Work out the finished part from the listing and answer in its coordinate system (mm). A direction names the side the tool comes from. Give positions to 0.01 mm unless a question says otherwise; leave off trailing zeros. Loops run counter-clockwise (first coordinate to the right, second up) from the corner with the lowest first, then second, coordinate; pieces in that order, holes last. Notation, with made-up numbers: (-22, 59.5) - (10, 59.5) arc R16 cw to (10, 88.5) - close; hole circle Ø9 at (38, 59). An arc over 180 degrees is marked (long way). Use CSV: the item, a comma, the result in double quotes.
Autodesk Inventor part; units mm, degrees
ref_plane "YZ Plane" through (0, 0, 0) normal (1, 0, 0) x (0, 1, 0)
ref_plane "XZ Plane" through (0, 0, 0) normal (0, 1, 0) x (-1, 0, 0)
ref_plane "XY Plane" through (0, 0, 0) normal (0, 0, 1) x (1, 0, 0)
sketch "Sketch1" plane through (0, 0, 0) normal (1, 0, 0) x (0, 1, 0)
  line L0 (10.236, 20.6024) -> (1.9777, 20.6024)
  line L1 (1.9777, 20.6024) -> (1.9777, 4.6508)
  line L2 (1.9777, 4.6508) -> (10.236, 4.6508)
  line L3 (10.236, 4.6508) -> (10.236, 20.6024)
  point P0 (0, 0)
extrude "Extrusion1" add sketch "Sketch1" along normal blind 25.4
sketch "Sketch2" plane through (0, 10.236, 20.6024) normal (0, 1, 0) x (1, 0, 0)
  line L0 (6.7613, 3.64) -> (20.9369, 3.64)
  line L1 (20.9369, 3.64) -> (20.9369, 12.1675)
  line L2 (20.9369, 12.1675) -> (6.7613, 12.1675)
  line L3 (6.7613, 12.1675) -> (6.7613, 3.64)
  line L4 (10.89, 6.1434) -> (17.4809, 6.1434)
  line L5 (17.4809, 6.1434) -> (17.4809, 9.7454)
  line L6 (17.4809, 9.7454) -> (11.2732, 9.7454)
  line L7 (11.2732, 9.7454) -> (11.2732, 6.1434)
  point P0 (0, 20.6024)
extrude "Extrusion2" add sketch "Sketch2" along normal blind 25.4 contours L3 L2 L1 L0 | L7 L6 L5 L4
sketch "Sketch3" plane through (0, 35.636, 20.6024) normal (0, 1, 0) x (1, 0, 0)
  line L0 (10.6145, 6.041) -> (18.3551, 6.041)
  line L1 (18.3551, 6.041) -> (18.3551, 10.1795)
  line L2 (18.3551, 10.1795) -> (10.6145, 10.1795)
  line L3 (10.6145, 10.1795) -> (10.6145, 6.041)
  point P0 (0, 20.6024)
extrude "Extrusion3" add sketch "Sketch3" along normal blind 25.4
properties part number "2nd model"
Item 1: Find the intervals of material crossed by line 1 (Y direction, x = 5.5, z = 12); line 2 (X direction, y = 23.5, z = 9.5); line 3 (Z direction, x = 8.75, y = 14.5), in increasing order.
Determined:
line 1,"y = 1.98 to 10.24"
line 2,"x = 6.76 to 20.94"
line 3,"z = 8.43 to 16.96"
Item 2: A cutting plane is placed at B-B on z = 12.5. Determine the outline of the cut face in (x, y), and give its area (3 significant figures).
Determined:
outline,"(0, 1.98) - (25.4, 1.98) - (25.4, 10.24) - (20.94, 10.24) - (20.94, 35.64) - (18.36, 35.64) - (18.36, 61.04) - (10.61, 61.04) - (10.61, 35.64) - (6.76, 35.64) - (6.76, 10.24) - (0, 10.24) - close"
area,"766 mm²"
Item 3: For faces 1 (the flat face through (14, 23, 16.962)), 2 (the flat face through (10.614, 48, 12)), 3 (the flat face through (14, 23, 8.435)), 4 (the flat face through (20.937, 23, 13)), determine the directions among +Z, -Z, +X, -X, +Y, -Y from which every point of the face is accessible in a straight line to the end or side of a thin tool.
Determined:
face 1,"+Z, +X, -X, +Y"
face 2,"+Z, -Z, -X, +Y"
face 3,"-Z, +X, -X, +Y"
face 4,"+Z, -Z, +X, +Y"
Item 4: A cutting plane is placed at C-C on y = 28. Determine the outline of the cut face in (x, z).
Determined:
outline,"(6.76, 8.43) - (20.94, 8.43) - (20.94, 16.96) - (6.76, 16.96) - close"
Item 5: A cutting plane is placed at A-A on x = 20. Determine the outline of the cut face in (y, z).
Determined:
outline,"(1.98, 4.65) - (10.24, 4.65) - (10.24, 8.43) - (35.64, 8.43) - (35.64, 16.96) - (10.24, 16.96) - (10.24, 20.6) - (1.98, 20.6) - close"
Item 6: A cutting plane is placed at D-D on x = 12. Determine the outline of the cut face in (y, z).
Determined:
outline,"(1.98, 4.65) - (10.24, 4.65) - (10.24, 8.43) - (35.64, 8.43) - (35.64, 10.42) - (61.04, 10.42) - (61.04, 14.56) - (35.64, 14.56) - (35.64, 16.96) - (10.24, 16.96) - (10.24, 20.6) - (1.98, 20.6) - close"
Item 7: Given P1, Ø2, axis at x = 12, y = 21, coming from the +Z side; P2, Ø4, axis at x = 14, y = 45.5, coming from the +Z side; P3, Ø2.5, axis at y = 18, z = 11.5, coming from the +X side, each flat-ended and moving along its own axis, determine where each tip first touches the part or whether it passes through.
Determined:
P1,"stops at z = 16.96"
P2,"stops at z = 14.56"
P3,"stops at x = 20.94"
